Autodesk Inventor part; units mm, degrees
ref_plane "工作平面1" through (0, -5.625, 0) normal (1, 0, 0) x (0, 0, -1)
ref_plane "YZ Plane" through (0, 0, 0) normal (1, 0, 0) x (0, 1, 0)
ref_plane "XZ Plane" through (0, 0, 0) normal (0, 1, 0) x (-1, 0, 0)
sketch "草图1" plane through (0, 0, 0) normal (0, 0, 1) x (1, 0, 0)
  line L0 (-6.475, -5.625) -> (6.475, -5.625)
  line L1 (6.475, -5.625) -> (6.475, 5.625)
  line L2 (6.475, 5.625) -> (-6.475, 5.625)
  line L3 (-6.475, 5.625) -> (-6.475, -5.625)
  line L4 (-6.475, -5.625) -> (6.475, 5.625) construction
  line L5 (6.475, -5.625) -> (-6.475, 5.625) construction
  line L6 (4.975, -4.225) -> (-4.975, -4.225)
  line L7 (-4.975, -4.225) -> (-4.975, 5.625)
  line L8 (-4.975, 5.625) -> (4.975, 5.625)
  line L9 (4.975, 5.625) -> (4.975, -4.225)
  line L10 (4.975, -4.225) -> (-4.975, 5.625) construction
  line L11 (-4.975, -4.225) -> (4.975, 5.625) construction
  line L12 (0, -7.875) -> (0, 7.875)
  point P0 (0, 0)
  point P1 (0, 0.7)
  point P2 (0, 0.7)
  dimension "d0" = 11.25
  dimension "d1" = 9.85
  dimension "d2" = 9.95
  dimension "d3" = 1.5
extrude "拉伸1" add sketch "草图1" along normal blind 11.5 contours L3 L2 L7 L6 L12 L0 | L12 L6 L9 L2 L1 L0
sketch "草图2" plane through (-6.475, -5.625, 0) normal (0, -1, 0) x (1, 0, 0)
  line L0 (0, 0) -> (12.95, 0)
  line L1 (12.95, 0) -> (12.95, 11.5)
  line L2 (0, 11.5) -> (12.95, 11.5)
  line L3 (0, 0) -> (0, 11.5)
  line L4 (0, 11.5) -> (12.95, 11.5) construction
  line L5 (6.475, 11.5) -> (6.475, 0) construction
  line L6 (12.95, 11.5) -> (11.45, 11.5) construction
  line L7 (12.95, 11.5) -> (14.65, 11.5)
  line L8 (12.95, 0) -> (12.95, 11.5) construction
  line L9 (12.95, 5.505) -> (14.65, 5.505)
  arc A0 (14.65, 5.505) -> (14.65, 11.5) centre (14.5281, 8.5025) ccw
  line L10 (0, 11.5) -> (-1.7, 11.5)
  line L11 (0, 5.505) -> (-1.7, 5.505)
  arc A1 (-1.7, 11.5) -> (-1.7, 5.505) centre (-1.5781, 8.5025) ccw
  point P0 (14.85, 8.55)
  point P1 (-1.9, 8.55)
  dimension "d6" = 1.7
  dimension "d7" = 3
  dimension "d8" = 1.9
  dimension "d9" = 2.95
extrude "拉伸2" add sketch "草图2" against normal blind 3.2 contours L1 L7 A0 L9
ref_plane "工作平面1" through (0, -5.625, 0) normal (1, 0, 0) x (0, 0, -1)
mirror "镜像1" about plane through (0, -5.625, 0) normal (1, 0, 0) of "拉伸2"
hole "孔1" at (8.375, -5.625, 8.55) at (-8.375, -5.625, 8.55) direction (0, 1, 0) diameter 3.2 end through all
fillet "圆角1" radius 1 2 edges at (4.975, -4.225, 5.75) (-4.975, -4.225, 5.75)
properties part number "N20电机座"
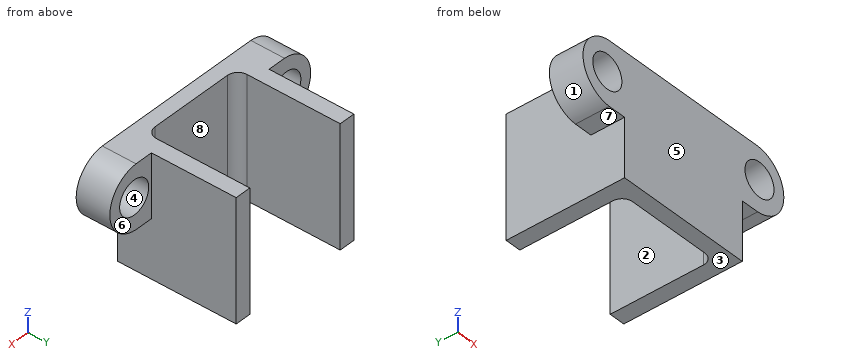
Source: CAD feature listing. Evaluate the final solid. Frame: model axes, mm. Face numbers are marked on the shaded views. A direction names the side the tool comes from. Coordinates: 2 decimals unless noted, no trailing zeros. Loops run counter-clockwise (first coordinate to the right, second up) from the corner with the lowest first, then second, coordinate; pieces in that order, holes last. Notation, with made-up numbers: M -37.5,-38.75 L 8.5,-38.75 A27 cw 8.5,-18.75 Z; hole C 76.5,36 d1. An arc over 180 degrees is marked long. Use CSV: the item, a comma, the result in double quotes.
(1) Cut plane A-A on y = 3. Return loops of the section in (x, z) (3 decimals), and give its area (3 significant figures).
Answers follow:
outline,"M -6.475,0 L -4.975,0 L -4.975,11.5 L -6.475,11.5 Z; M 4.975,0 L 6.475,0 L 6.475,11.5 L 4.975,11.5 Z"
area,"34.5 mm²"
(2) Cut plane D-D on x = -1. Return loops of the section in (y, z) (3 decimals), and give its area (3 significant figures).
Answers follow:
outline,"M -5.625,0 L -4.225,0 L -4.225,11.5 L -5.625,11.5 Z"
area,"16.1 mm²"
(3) Contact query for flat-ended pins moving along their axis: pin 1 (2.5 mm diameter, centred on x = -8, z = 8, fed in from +Y) (3 decimals); pin 2 (5 mm diameter, centred on y = 3, z = 6, fed in from +X) (3 decimals); pin 3 (4 mm diameter, centred on x = -1.5, z = 8, fed in from +Y) (3 decimals). Output: stop coordinate, or through.
Answers follow:
pin 1,"y = -2.425"
pin 2,"x = 6.475"
pin 3,"y = -4.225"
(4) Cut plane B-B on z = 8.75. Return loops of the section in (x, y) (3 decimals).
Answers follow:
outline,"M -11.043,-5.625 L -9.962,-5.625 L -9.962,-2.425 L -11.043,-2.425 Z; M -6.788,-5.625 L 6.788,-5.625 L 6.788,-2.425 L 6.475,-2.425 L 6.475,5.625 L 4.975,5.625 L 4.975,-3.225 A1 cw 3.975,-4.225 L -3.975,-4.225 A1 cw -4.975,-3.225 L -4.975,5.625 L -6.475,5.625 L -6.475,-2.425 L -6.788,-2.425 Z; M 9.962,-5.625 L 11.043,-5.625 L 11.043,-2.425 L 9.962,-2.425 Z"
(5) Draft query along Z for the marked faces 1, 2, 3 and 4. Return one class per face: pulls with the +Z half, pulls with the -Z half, needs draft (parallel to the pull), parting line crosses it, or undercut.
Answers follow:
face 1,"parting line crosses it"
face 2,"needs draft"
face 3,"pulls with the -Z half"
face 4,"undercut"
(6) Reachability of the marked faces 5, 6, 7 and 8 from +Z, -Z, +X, -X, +Y, -Y: full face, straight path, thin tool, end or side. Return the list, or none.
Answers follow:
face 5,"+Z, -Z, +X, -X, -Y"
face 6,"+Z, -Z, +X, +Y"
face 7,"-Z, -X, +Y, -Y"
face 8,"+Z, -Z, +Y"
(7) Line query: line 1 (X direction, y = -4.4, z = 8.55) (3 decimals); line 2 (X direction, y = 3.75, z = 7.75) (3 decimals); line 3 (X direction, y = -3.7, z = 8.55) (3 decimals). Output: solid intervals per line, ascending. Write a range as [from, to].
Answers follow:
line 1,"[-11.053, -9.975], [-6.775, 6.775], [9.975, 11.053]"
line 2,"[-6.475, -4.975], [4.975, 6.475]"
line 3,"[-11.053, -9.975], [-6.775, -4.855], [4.855, 6.775], [9.975, 11.053]"
(8) Cut plane C-C on z = 3.5. Return loops of the section in (x, y) (3 decimals).
Answers follow:
outline,"M -6.475,-5.625 L 6.475,-5.625 L 6.475,5.625 L 4.975,5.625 L 4.975,-3.225 A1 cw 3.975,-4.225 L -3.975,-4.225 A1 cw -4.975,-3.225 L -4.975,5.625 L -6.475,5.625 Z"
